```python
from build123d import *

# Parameters (mm, degrees)
F0_W     = 100.364631
F0_H     = 200.412475
F1_DEPTH = 5
F2_W     = 50.194541
F2_H     = 40.442418
F3_DEPTH = 25
F5_D     = 25


with BuildPart() as f1:
    # F0 (on Top) → F1 (new body)
    with BuildSketch(Plane.XY):
        with Locations((-26.610498, -24.112809)):
            Rectangle(F0_W, F0_H)
    extrude(amount=F1_DEPTH)

    # F2 (on face) → F3 (join)
    with BuildSketch(Plane.XY.offset(5)):
        with Locations((-51.695543, 55.872219)):
            Rectangle(F2_W, F2_H)
    extrude(amount=F3_DEPTH)

    # F5 (through all)
    with Locations(Plane.XY.offset(5)):
        with Locations((-11.947709, -94.156161)):
            Hole(F5_D / 2)


solid = f1.part
```
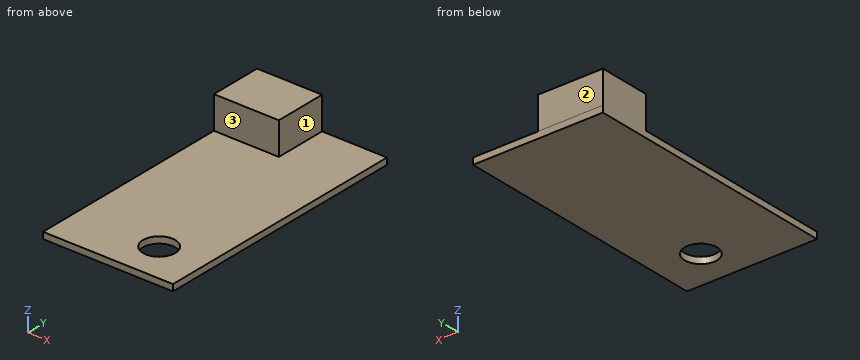
Work out the finished part from the listing and answer in its coordinate system (mm). Face numbers are marked on the shaded views. A direction names the side the tool comes from. Coordinates: 2 decimals unless noted, no trailing zeros. Loops run counter-clockwise (first coordinate to the right, second up) from the corner with the lowest first, then second, coordinate; pieces in that order, holes last. Notation, with made-up numbers: M 73.25,47.25 L 131.25,47.25 A17 ccw 131.25,78.25 Z; hole C 83,5.25 d4. An arc over 180 degrees is marked long. Use CSV: the item, a comma, the result in double quotes. Start each with the question number.
(1) Find section D-D, the plane z = 22.5. Give the vertices of the cut face in (x, y).
(2) For the marked faces 1, 2 and 3, determine the directions among +Z, -Z, +X, -X, +Y, -Y from which every point of the face is accessible in a straight line to the end or side of a thin tool.
(3) Given pin 1 Ø1 at (x, z) = (-27, 25.5) entering from -Y; pin 2 Ø10 at (x, y) = (2.5, 29.5) entering from +Z; pin 3 Ø7.5 at (y, z) = (48.5, 22) entering from +X, each flat-ended and moving along its own axis, determine where each tip first touches the part or whether it passes through.
(4) Find section C-C, the plane y = 31. Give the vertices of the cut face in (x, z).
(5) Find section A-A, the plane x = -37.5. Give the vertices of the cut face in (y, z), then the cut area to 3 significant figures.
(6) Consider line 1 (X direction, y = 55.5, z = 6.75); line 2 (Z direction, x = -14, y = -72.5); line 3 (Y direction, x = -59.5, z = 17). Determine where each line is inside the solid, lowest interval first.
(7) Find section B-B, the plane z = 2.5. Give the vertices of the cut face in (x, y), then the cut area to 3 significant figures.
Recorded:
1,outline,"M -76.79,35.65 L -26.6,35.65 L -26.6,76.09 L -76.79,76.09 Z"
2,face 1,"+Z, +X, +Y, -Y"
2,face 2,"+Z, -Z, +X, -X, +Y"
2,face 3,"+Z, +X, -X, -Y"
3,pin 1,"stops at y = 35.65"
3,pin 2,"stops at z = 5"
3,pin 3,"stops at x = -26.6"
4,outline,"M -76.79,0 L 23.57,0 L 23.57,5 L -76.79,5 Z"
5,outline,"M -124.32,0 L 76.09,0 L 76.09,30 L 35.65,30 L 35.65,5 L -124.32,5 Z"
5,area,"2,010 mm^2"
6,line 1,"x = -76.79 to -26.6"
6,line 2,"z = 0 to 5"
6,line 3,"y = 35.65 to 76.09"
7,outline,"M -76.79,-124.32 L 23.57,-124.32 L 23.57,76.09 L -76.79,76.09 Z; hole C -11.95,-94.16 d25"
7,area,"19,600 mm^2"
